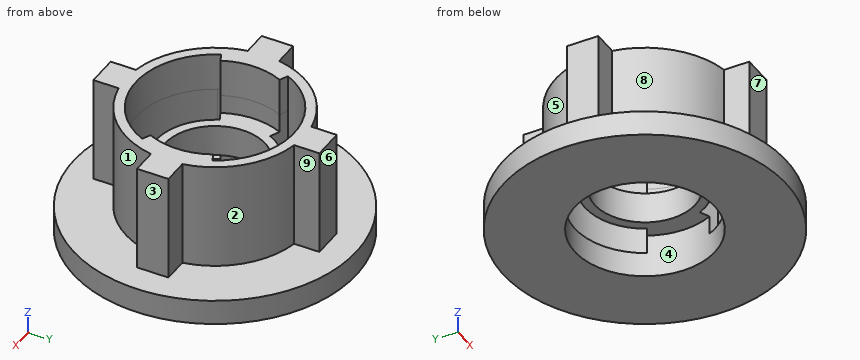
from build123d import *
from build123d.topology import SkipClean

# Parameters (mm, degrees)
ESBO_O1_R                 = 11.15
RESSALTO_EXTRUS_O1_DEPTH  = 15
ESBO_O2_R                 = 22.5
RESSALTO_EXTRUS_O2_DEPTH  = 4
RESSALTO_EXTRUS_O6_START  = -8
ESBO_O5_R                 = 11.15
ESBO_O5_R_2               = 8
RESSALTO_EXTRUS_O6_DEPTH  = 8
RESSALTO_EXTRUS_O7_START  = 4
ESBO_O7_R                 = 14.2
ESBO_O7_R_2               = 11.15
RESSALTO_EXTRUS_O7_DEPTH  = 4
RESSALTO_EXTRUS_O8_START  = 4
ESBO_O8_R                 = 11.15
ESBO_O8_R_2               = 8
RESSALTO_EXTRUS_O8_DEPTH  = 4
CORTE_EXTRUS_O1_DEPTH     = 7
CORTE_EXTRUS_O2_DEPTH     = 8
CORTE_EXTRUS_O3_START     = -4
CORTE_EXTRUS_O3_DEPTH     = 4
CORTE_EXTRUS_O4_START     = -11
CORTE_EXTRUS_O4_DEPTH     = 11
CORTE_EXTRUS_O5_START     = -3
ESBO_O17_R                = 11.15
CORTE_EXTRUS_O5_DEPTH     = 3
RESSALTO_EXTRUS_O11_DEPTH = 6


with BuildPart() as part:
    # Esbo_o1 → Ressalto-extrus_o1 (new body)
    with BuildSketch(Plane.XY):
        with BuildLine():
            Line((-2.5, 18), (-2.5, 13.978197309))
            ThreePointArc((-2.5, 13.978197309), (-10.040916293, 10.040916293), (-13.978197309, 2.5))
            Line((-13.978197309, 2.5), (-18, 2.5))
            Line((-18, 2.5), (-18, -2.5))
            Line((-18, -2.5), (-13.978197309, -2.5))
            ThreePointArc((-13.978197309, -2.5), (-10.040916293, -10.040916293), (-2.5, -13.978197309))
            Line((-2.5, -13.978197309), (-2.5, -18))
            Line((-2.5, -18), (2.5, -18))
            Line((2.5, -18), (2.5, -13.978197309))
            ThreePointArc((2.5, -13.978197309), (10.040916293, -10.040916293), (13.978197309, -2.5))
            Line((13.978197309, -2.5), (18, -2.5))
            Line((18, -2.5), (18, 2.5))
            Line((18, 2.5), (13.978197309, 2.5))
            ThreePointArc((13.978197309, 2.5), (10.040916293, 10.040916293), (2.5, 13.978197309))
            Line((2.5, 13.978197309), (2.5, 18))
            Line((2.5, 18), (-2.5, 18))
        make_face()
        Circle(ESBO_O1_R, mode=Mode.SUBTRACT)
    extrude(amount=RESSALTO_EXTRUS_O1_DEPTH)

    # Esbo_o5 → Ressalto-extrus_o6 (add)
    with BuildSketch(Plane.XY.offset(15).offset(RESSALTO_EXTRUS_O6_START)):
        Circle(ESBO_O5_R)
        Circle(ESBO_O5_R_2, mode=Mode.SUBTRACT)
    extrude(amount=RESSALTO_EXTRUS_O6_DEPTH)



with BuildPart() as body_2:
    # Esbo_o2 → Ressalto-extrus_o2 (new body)
    # profile 1 of 5: a face of its own
    with SkipClean():  # the faces are left unmerged after this step: merging them gives an invalid solid
        with BuildSketch(Plane(origin=(0, 0, 0), x_dir=(-1, 0, 0), z_dir=(0, 0, -1))):
            Circle(ESBO_O2_R)
            with BuildLine():
                Line((2.5, 13.978197309), (2.5, 18))
                Line((2.5, 18), (-2.5, 18))
                Line((-2.5, 18), (-2.5, 13.978197309))
                ThreePointArc((-2.5, 13.978197309), (-10.040916293, 10.040916293), (-13.978197309, 2.5))
                Line((-13.978197309, 2.5), (-18, 2.5))
                Line((-18, 2.5), (-18, -2.5))
                Line((-18, -2.5), (-13.978197309, -2.5))
                ThreePointArc((-13.978197309, -2.5), (-10.040916293, -10.040916293), (-2.5, -13.978197309))
                Line((-2.5, -13.978197309), (-2.5, -18))
                Line((-2.5, -18), (2.5, -18))
                Line((2.5, -18), (2.5, -13.978197309))
                ThreePointArc((2.5, -13.978197309), (10.040916293, -10.040916293), (13.978197309, -2.5))
                Line((13.978197309, -2.5), (18, -2.5))
                Line((18, -2.5), (18, 2.5))
                Line((18, 2.5), (13.978197309, 2.5))
                ThreePointArc((13.978197309, 2.5), (10.040916293, 10.040916293), (2.5, 13.978197309))
            make_face(mode=Mode.SUBTRACT)
        # profile 2 of 5: a face of its own
        with BuildSketch(Plane(origin=(0, 0, 0), x_dir=(-1, 0, 0), z_dir=(0, 0, -1))):
            with BuildLine():
                Line((2.5, -18), (2.5, -13.978197309))
                ThreePointArc((2.5, -13.978197309), (0, -14.2), (-2.5, -13.978197309))
                Line((-2.5, -13.978197309), (-2.5, -18))
                Line((-2.5, -18), (2.5, -18))
            make_face()
        # profile 3 of 5: a face of its own
        with BuildSketch(Plane(origin=(0, 0, 0), x_dir=(-1, 0, 0), z_dir=(0, 0, -1))):
            with BuildLine():
                ThreePointArc((-13.978197309, -2.5), (-14.2, 0), (-13.978197309, 2.5))
                Line((-13.978197309, 2.5), (-18, 2.5))
                Line((-18, 2.5), (-18, -2.5))
                Line((-18, -2.5), (-13.978197309, -2.5))
            make_face()
        # profile 4 of 5: a face of its own
        with BuildSketch(Plane(origin=(0, 0, 0), x_dir=(-1, 0, 0), z_dir=(0, 0, -1))):
            with BuildLine():
                ThreePointArc((-2.5, 13.978197309), (0, 14.2), (2.5, 13.978197309))
                Line((2.5, 13.978197309), (2.5, 18))
                Line((2.5, 18), (-2.5, 18))
                Line((-2.5, 18), (-2.5, 13.978197309))
            make_face()
        # profile 5 of 5: a face of its own
        with BuildSketch(Plane(origin=(0, 0, 0), x_dir=(-1, 0, 0), z_dir=(0, 0, -1))):
            with BuildLine():
                Line((18, 2.5), (13.978197309, 2.5))
                ThreePointArc((13.978197309, 2.5), (14.2, 0), (13.978197309, -2.5))
                Line((13.978197309, -2.5), (18, -2.5))
                Line((18, -2.5), (18, 2.5))
            make_face()
        extrude(amount=RESSALTO_EXTRUS_O2_DEPTH)


with BuildPart() as part_1:
    with SkipClean():  # the faces are left unmerged after this step: merging them gives an invalid solid
        add(part.part)

        add(body_2.part)  # Ressalto-extrus_o7 merges body 2
        # Esbo_o7 → Ressalto-extrus_o7 (add)
        with BuildSketch(Plane(origin=(0, 0, 0), x_dir=(-1, 0, 0), z_dir=(0, 0, -1)).offset(RESSALTO_EXTRUS_O7_START)):
            Circle(ESBO_O7_R)
            with Locations(Location((0, 0, 0), (0, 0, 180))):
                Circle(ESBO_O7_R_2, mode=Mode.SUBTRACT)
        extrude(amount=-RESSALTO_EXTRUS_O7_DEPTH)

    # Esbo_o8 → Ressalto-extrus_o8 (add)
    with BuildSketch(Plane(origin=(0, 0, 7), x_dir=(-1, 0, 0), z_dir=(0, 0, -1)).offset(RESSALTO_EXTRUS_O8_START)):
        Circle(ESBO_O8_R)
        with Locations(Location((0, 0, 0), (0, 0, 180))):
            Circle(ESBO_O8_R_2, mode=Mode.SUBTRACT)
    extrude(amount=-RESSALTO_EXTRUS_O8_DEPTH)

    # Esbo_o11 → Corte-extrus_o1 (cut)
    with BuildSketch(Plane.XY.offset(15)):
        with BuildLine():
            Line((-11.191152491, -5.789482353), (-8.437773704, -4.365085901))
            ThreePointArc((-8.437773704, -4.365085901), (0.195118203, -9.497996046), (8.609923977, -4.014873487))
            Line((8.609923977, -4.014873487), (11.419478117, -5.324990098))
            ThreePointArc((11.419478117, -5.324990098), (0.258788353, -12.597342124), (-11.191152491, -5.789482353))
        make_face()
        with BuildLine():
            Line((-11.419478117, 5.324990098), (-8.609923977, 4.014873487))
            ThreePointArc((-8.609923977, 4.014873487), (-0.195118203, 9.497996046), (8.437773704, 4.365085901))
            Line((8.437773704, 4.365085901), (11.191152491, 5.789482353))
            ThreePointArc((11.191152491, 5.789482353), (-0.258788353, 12.597342124), (-11.419478117, 5.324990098))
        make_face()
    extrude(amount=-CORTE_EXTRUS_O1_DEPTH, mode=Mode.SUBTRACT)

    # Esbo_o12 → Corte-extrus_o2 (cut)
    with BuildSketch(Plane.XY.offset(8)):
        with BuildLine():
            Line((11.419478117, -5.324990098), (8.609923977, -4.014873487))
            ThreePointArc((8.609923977, -4.014873487), (0.195118203, -9.497996046), (-8.437773704, -4.365085901))
            Line((-8.437773704, -4.365085901), (-11.191152491, -5.789482353))
            ThreePointArc((-11.191152491, -5.789482353), (0.258788353, -12.597342124), (11.419478117, -5.324990098))
        make_face()
        with BuildLine():
            Line((-11.419478117, 5.324990098), (-8.609923977, 4.014873487))
            ThreePointArc((-8.609923977, 4.014873487), (-0.195118203, 9.497996046), (8.437773704, 4.365085901))
            Line((8.437773704, 4.365085901), (11.191152491, 5.789482353))
            ThreePointArc((11.191152491, 5.789482353), (-0.258788353, 12.597342124), (-11.419478117, 5.324990098))
        make_face()
    extrude(amount=-CORTE_EXTRUS_O2_DEPTH, mode=Mode.SUBTRACT)

    # Esbo_o13 → Corte-extrus_o3 (cut)
    with BuildSketch(Plane.XY.offset(15).offset(CORTE_EXTRUS_O3_START)):
        with BuildLine():
            Line((-2.5, 18), (-2.5, 13.978197309))
            ThreePointArc((-2.5, 13.978197309), (-10.040916293, 10.040916293), (-13.978197309, 2.5))
            Line((-13.978197309, 2.5), (-18, 2.5))
            Line((-18, 2.5), (-18, -2.5))
            Line((-18, -2.5), (-13.978197309, -2.5))
            ThreePointArc((-13.978197309, -2.5), (-10.040916293, -10.040916293), (-2.5, -13.978197309))
            Line((-2.5, -13.978197309), (-2.5, -18))
            Line((-2.5, -18), (2.5, -18))
            Line((2.5, -18), (2.5, -13.978197309))
            ThreePointArc((2.5, -13.978197309), (10.040916293, -10.040916293), (13.978197309, -2.5))
            Line((13.978197309, -2.5), (18, -2.5))
            Line((18, -2.5), (18, 2.5))
            Line((18, 2.5), (13.978197309, 2.5))
            ThreePointArc((13.978197309, 2.5), (10.040916293, 10.040916293), (2.5, 13.978197309))
            Line((2.5, 13.978197309), (2.5, 18))
            Line((2.5, 18), (-2.5, 18))
        make_face()
    extrude(amount=CORTE_EXTRUS_O3_DEPTH, mode=Mode.SUBTRACT)

    # Esbo_o14 → Corte-extrus_o4 (cut)
    with BuildSketch(Plane.XY.offset(11).offset(CORTE_EXTRUS_O4_START)):
        with BuildLine():
            Line((11.191152491, 5.789482353), (8.437773704, 4.365085901))
            ThreePointArc((8.437773704, 4.365085901), (-0.195118203, 9.497996046), (-8.609923977, 4.014873487))
            Line((-8.609923977, 4.014873487), (-11.419478117, 5.324990098))
            ThreePointArc((-11.419478117, 5.324990098), (-0.258788353, 12.597342124), (11.191152491, 5.789482353))
        make_face()
        with BuildLine():
            Line((-8.609923977, -4.014873487), (-11.419478117, -5.324990098))
            ThreePointArc((-11.419478117, -5.324990098), (-11.307700579, -5.55840873), (-11.191152491, -5.789482353))
            Line((-11.191152491, -5.789482353), (-8.437773704, -4.365085901))
            ThreePointArc((-8.437773704, -4.365085901), (-8.525647262, -4.190863725), (-8.609923977, -4.014873487))
        make_face()
    extrude(amount=CORTE_EXTRUS_O4_DEPTH, mode=Mode.SUBTRACT)

    # Esbo_o17 → Corte-extrus_o5 (cut)
    with SkipClean():  # the faces are left unmerged after this step: merging them gives an invalid solid
        with BuildSketch(Plane.XY.offset(11).offset(CORTE_EXTRUS_O5_START)):
            with Locations(Location((0, 0, 0), (0, 0, 335))):
                Circle(ESBO_O17_R)
        extrude(amount=CORTE_EXTRUS_O5_DEPTH, mode=Mode.SUBTRACT)

    # Esbo_o18 → Ressalto-extrus_o11 (add)
    with SkipClean():  # the faces are left unmerged after this step: merging them gives an invalid solid
        with BuildSketch(Plane.XY.offset(11)):
            with BuildLine():
                Line((2.5, 13.978197309), (2.5, 18))
                Line((2.5, 18), (-2.5, 18))
                Line((-2.5, 18), (-2.5, 13.978197309))
                ThreePointArc((-2.5, 13.978197309), (-10.040916293, 10.040916293), (-13.978197309, 2.5))
                Line((-13.978197309, 2.5), (-18, 2.5))
                Line((-18, 2.5), (-18, -2.5))
                Line((-18, -2.5), (-13.978197309, -2.5))
                ThreePointArc((-13.978197309, -2.5), (-10.040916293, -10.040916293), (-2.5, -13.978197309))
                Line((-2.5, -13.978197309), (-2.5, -18))
                Line((-2.5, -18), (2.5, -18))
                Line((2.5, -18), (2.5, -13.978197309))
                ThreePointArc((2.5, -13.978197309), (10.040916293, -10.040916293), (13.978197309, -2.5))
                Line((13.978197309, -2.5), (18, -2.5))
                Line((18, -2.5), (18, 2.5))
                Line((18, 2.5), (13.978197309, 2.5))
                ThreePointArc((13.978197309, 2.5), (10.040916293, 10.040916293), (2.5, 13.978197309))
            make_face()
            with BuildLine():
                Line((-11.419478117, -5.324990098), (-10.105331825, -4.712193618))
                ThreePointArc((-10.105331825, -4.712193618), (-11.15, 0), (-10.105331825, 4.712193618))
                Line((-10.105331825, 4.712193618), (-11.419478117, 5.324990098))
                ThreePointArc((-11.419478117, 5.324990098), (-0.258788353, 12.597342124), (11.191152491, 5.789482353))
                Line((11.191152491, 5.789482353), (9.903281768, 5.1232324))
                ThreePointArc((9.903281768, 5.1232324), (11.147647991, 0.229007154), (10.105331825, -4.712193618))
                Line((10.105331825, -4.712193618), (11.419478117, -5.324990098))
                ThreePointArc((11.419478117, -5.324990098), (0, -12.6), (-11.419478117, -5.324990098))
            make_face(mode=Mode.SUBTRACT)
        extrude(amount=RESSALTO_EXTRUS_O11_DEPTH)


solid = part_1.part
CAD build for the part. Positions are in the model's coordinates, mm. Face numbers are marked on the shaded views. A direction names the side the tool comes from. Give positions to 0.01 mm unless a question says otherwise; leave off trailing zeros. Write each loop counter-clockwise with the first axis right and the second up, starting at its lowest first coordinate (ties: lowest second). Pieces come first, ordered by that corner, then holes. Notation, with made-up numbers: M 8.5,8.25 L 21.5,8.25 A22 ccw 21.5,38.25 Z; hole C 64,20 d1. An arc over 180 degrees is marked long. Put each result on its own line as item: value. Start each with the question number.
(1) Mould opens along Y. For the marked faces 1, 2, 3 and 4 say: +Y half, -Y half, draft (parallel to the pull), parting line (faces both ways), or undercut.
(2) Band-saw the part on B-B, the plane z = 9. Write the cut outline in (x, y) (3 decimals), and give its area (3 significant figures).
(3) Band-saw the part on A-A, the plane y = 0. Write the cut outline in (x, z).
(4) Which spindle directions (+Z, -Z, +X, -X, +Y, -Y) get a long thin tool onto all of the face, cutting with end or side? Do the marked faces 5, 6, 7, 8 and 9. Say none if no direction does.
(5) Band-saw the part on D-D, the plane z = 5. Write the cut outline in (x, y) (3 decimals), and give its area (3 significant figures).
(6) Flat gauge pins, fed straight in: pin 1 Ø1.5 at (x, z) = (6, -1) entering from -Y; pin 2 Ø2 at (y, z) = (-16, 5.5) entering from -X; pin 3 Ø3 at (x, z) = (-1, 1) entering from +Y. Where does each tip first touch, or does it go through?
(7) Band-saw the part on C-C, the plane x = 5. Write the cut outline in (y, z) (3 decimals), and give its area (3 significant figures).
(8) Probe L1, parallel to Y at x = 0, z = 4.4; L2, parallel to Y at x = 0, z = -2; L3, parallel to Y at x = 0, z = 0.25. List the from-to ranges inside material, lowest first.
Response values:
1. face 1: -Y half
1. face 2: +Y half
1. face 3: draft
1. face 4: undercut
2. outline: M -18,-2.5 L -13.978,-2.5 A14.2 ccw -2.5,-13.978 L -2.5,-18 L 2.5,-18 L 2.5,-13.978 A14.2 ccw 13.978,-2.5 L 18,-2.5 L 18,2.5 L 13.978,2.5 A14.2 ccw 2.5,13.978 L 2.5,18 L -2.5,18 L -2.5,13.978 A14.2 ccw -13.978,2.5 L -18,2.5 Z; hole M -11.419,-5.325 A12.6 ccw -11.191,-5.789 A12.6 ccw 11.419,-5.325 L 10.105,-4.712 A11.15 ccw 9.903,5.123 L 11.191,5.789 A12.6 ccw -11.419,5.325 L -10.105,4.712 A11.15 ccw -10.105,-4.712 Z
2. area: 243 mm2
3. outline: M -22.5,-4 L -11.15,-4 L -11.15,3 L -8,3 L -8,8 L -11.15,8 L -11.15,17 L -18,17 L -18,0 L -22.5,0 Z; M 8,3 L 11.15,3 L 11.15,-4 L 22.5,-4 L 22.5,0 L 18,0 L 18,17 L 11.15,17 L 11.15,8 L 8,8 Z
4. face 5: +Z, -X, +Y
4. face 6: +Z, +X, -X, +Y
4. face 7: +Z, +X, -X, -Y
4. face 8: +Z, -X, -Y
4. face 9: +Z, +X, +Y
5. outline: M -18,-2.5 L -13.978,-2.5 A14.2 ccw -2.5,-13.978 L -2.5,-18 L 2.5,-18 L 2.5,-13.978 A14.2 ccw 13.978,-2.5 L 18,-2.5 L 18,2.5 L 13.978,2.5 A14.2 ccw 2.5,13.978 L 2.5,18 L -2.5,18 L -2.5,13.978 A14.2 ccw -13.978,2.5 L -18,2.5 Z; hole M -11.419,-5.325 A12.6 ccw -11.191,-5.789 A12.6 ccw 11.419,-5.325 L 8.61,-4.015 A9.5 cw -8.438,-4.365 A9.5 cw -8.61,-4.015 Z; hole M -11.419,5.325 L -8.61,4.015 A9.5 cw 8.438,4.365 L 11.191,5.789 A12.6 ccw Z; hole C 0,0 d16
5. area: 356 mm2
6. pin 1: stops at y = -21.88
6. pin 2: stops at x = -2.5
6. pin 3: stops at y = 22.5
7. outline: M -21.937,-4 L -9.966,-4 L -9.966,0 L -11.565,0 L -11.565,17 L -13.291,17 L -13.291,0 L -21.937,0 Z; M -8.078,3 L -6.245,3 L -6.245,8 L -8.078,8 Z; M 6.245,3 L 8.078,3 L 8.078,8 L 6.245,8 Z; M 9.966,-4 L 21.937,-4 L 21.937,0 L 13.291,0 L 13.291,17 L 11.565,17 L 11.565,0 L 9.966,0 Z
7. area: 173 mm2
8. L1: y = -18 to -12.6, -9.5 to -8, 8 to 9.5, 12.6 to 18
8. L2: y = -22.5 to -11.15, 11.15 to 22.5
8. L3: y = -18 to -12.6, 12.6 to 18
